Check sheet for the modelled part. Datum: model origin and axes. Units: mm. A direction names the side the tool comes from. Round coordinates to 2 decimals unless told otherwise and drop trailing zeros. Loops run counter-clockwise (first coordinate to the right, second up) from the corner with the lowest first, then second, coordinate; pieces in that order, holes last. Notation, with made-up numbers: (10.5, 48.5) -> (29.5, 48.5) arc R24 ccw to (29.5, 77.5) -> close; hole circle Ø9 at (31, 83). An arc over 180 degrees is marked (long way). Use one line per item in the form item = value. Start each with the question number.
(1) Go/stop test with flat-tipped pins: pin 1 (1.5 mm diameter, centred on x = -499, z = -663, fed in from +Y); pin 2 (2 mm diameter, centred on x = -357, y = 1222, fed in from +Z); pin 3 (12 mm diameter, centred on x = -530.68, z = -637.45, fed in from +Y); pin 4 (3 mm diameter, centred on x = -415, y = 993, fed in from -Z). Record where each tip stops, or that it passes through.
(2) Set-up check for faces 4 (the flat face through (-446, 1069, -657.097)), 5 (the cylindrical face through (-394.39, 1308.86, -642.06)), 6 (the flat face through (-486, 883, -732.097)), 7 (the flat face through (-404, 1075.621, -637)), 8 (the flat face through (-486, 873.179, -674)): record each of +Z, -Z, +X, -X, +Y, -Y from which the full face is reachable in a straight line by a thin tool's end or side.
(3) Sectioned sample at A-A (x = -366). Record the cut outline in (y, z).
(4) Draft check along X on faces 1 (the flat face through (-486, 893.179, -694)), 2 (the flat face through (-531, 926.127, -637)), 3 (the flat face through (-666.625, 1090, -641)). Enter one of: released by +X, released by -X, zero draft, split by the parting line, or undercut.
(5) Sectioned sample at B-B (y = 964.5). Record the cut outline in (x, z), and give its area (3 significant figures).
(6) Sectioned sample at C-C (y = 1179). Record the cut outline in (x, z), and give its area (3 significant figures).
(7) Sectioned sample at D-D (z = -634). Record the cut outline in (x, y).
(8) Material ranges on probe 1 along X at (y, z) = (1170.5, -637.5); probe 2 along Y at (x, z) = (-546, -626); probe 3 along X at (y, z) = (1058.5, -638), recorded low to high. Write a range as [from, to].
from build123d import *

# Parameters (mm, degrees)
SKETCH_1_W                      = 365.93
SKETCH_1_H                      = 455
SKETCH_1_R                      = 10
SKETCH_1_R_2                    = 14.438127561
SKETCH_1_W_2                    = 96.91
SKETCH_1_H_2                    = 352.59
SKETCH_1_H_3                    = 203.096012828
EXTRUDE_1_DEPTH                 = 40.26
CUT_EXTRUDE_1_REACH             = 1042.764
SKETCH_2_R                      = 10
CUT_EXTRUDE_1_DIRECTION_2_DEPTH = 1041.76399807
SKETCH_3_W                      = 365.93
SKETCH_3_H                      = 20
EXTRUDE_2_DEPTH                 = 80
CUT_EXTRUDE_2_REACH             = 1086.862
SKETCH_6_R                      = 12.5
CUT_EXTRUDE_4_DEPTH             = 1571.967331718
CUT_EXTRUDE_4_DEPTH_BACK        = 1571.967331718
SKETCH_9_W                      = 5
SKETCH_9_H                      = 20
CUT_EXTRUDE_5_DEPTH             = 1569.627549285
CUT_EXTRUDE_5_DEPTH_BACK        = 1569.627549285
SKETCH_10_W                     = 75
SKETCH_10_H                     = 10
SKETCH_11_W                     = 365.93
SKETCH_11_H                     = 115.26
SKETCH_11_R                     = 12.5
EXTRUDE_4_DEPTH                 = 10


with BuildPart() as part:
    # 草图1 → 凸台-拉伸1 (new body)
    with BuildSketch(Plane.XY.offset(-616.836895005)):
        with Locations((-483.659609698, 1110.678523142)):
            Rectangle(SKETCH_1_W, SKETCH_1_H)
        with Locations((-607.210787573, 1138.804962693)):
            Circle(SKETCH_1_R, mode=Mode.SUBTRACT)
        with Locations((-403.264609698, 1019.178523142)):
            Circle(SKETCH_1_R_2, mode=Mode.SUBTRACT)
        with Locations((-530.676153664, 1102.421638316)):
            Rectangle(SKETCH_1_W_2, SKETCH_1_H_2, mode=Mode.SUBTRACT)
        with Locations((-403.264609698, 1177.168631902)):
            Rectangle(SKETCH_1_W_2, SKETCH_1_H_3, mode=Mode.SUBTRACT)
    extrude(amount=-EXTRUDE_1_DEPTH)

    # 草图2 → 切除-拉伸1 (cut, up to next)
    with BuildSketch(Plane(origin=(0, 1338.178523142, 0), x_dir=(1, 0, 0), z_dir=(0, 1, 0)), mode=Mode.PRIVATE) as cut_extrude_1_sk1:
        with Locations(Location((-530.676153664, 637.446895005, 0), (0, 0, 90))):
            Circle(SKETCH_2_R)
    cut_extrude_1_tool1 = extrude(cut_extrude_1_sk1.sketch, amount=-CUT_EXTRUDE_1_REACH, mode=Mode.PRIVATE) & part.part
    # 草图2 → 切除-拉伸1 (cut, up to next)
    with BuildSketch(Plane(origin=(0, 1338.178523142, 0), x_dir=(1, 0, 0), z_dir=(0, 1, 0)), mode=Mode.PRIVATE) as cut_extrude_1_sk2:
        with Locations(Location((-403.264609698, 637.446895005, 0), (0, 0, 90))):
            Circle(SKETCH_2_R)
    cut_extrude_1_tool2 = extrude(cut_extrude_1_sk2.sketch, amount=-CUT_EXTRUDE_1_REACH, mode=Mode.PRIVATE) & part.part
    add(cut_extrude_1_tool1.solids().sort_by_distance((-530.676154, 1338.178523, -637.446895))[0], mode=Mode.SUBTRACT)
    add(cut_extrude_1_tool2.solids().sort_by_distance((-403.26461, 1338.178523, -637.446895))[0], mode=Mode.SUBTRACT)

    # 草图2 → 切除-拉伸1 direction 2 (cut)
    with BuildSketch(Plane(origin=(0, 1338.178523142, 0), x_dir=(1, 0, 0), z_dir=(0, 1, 0))):
        with Locations(Location((-530.676153664, 637.446895005, 0), (0, 0, 90))):
            Circle(SKETCH_2_R)
        with Locations(Location((-403.264609698, 637.446895005, 0), (0, 0, 90))):
            Circle(SKETCH_2_R)
    extrude(amount=CUT_EXTRUDE_1_DIRECTION_2_DEPTH, mode=Mode.SUBTRACT)

    # 草图3 → 凸台-拉伸2 (add)
    with BuildSketch(Plane(origin=(0, 0, -657.096895005), x_dir=(-1, 0, 0), z_dir=(0, 0, -1))):
        with Locations((483.659609698, 893.178523142)):
            Rectangle(SKETCH_3_W, SKETCH_3_H)
    extrude(amount=EXTRUDE_2_DEPTH)

    # 草图6 → 切除-拉伸2 (cut, up to next)
    with BuildSketch(Plane(origin=(0, 903.178523142, 0), x_dir=(1, 0, 0), z_dir=(0, 1, 0)), mode=Mode.PRIVATE) as cut_extrude_2_sk1:
        with Locations(Location((-566.624609698, 697.096895005, 0), (0, 0, 270))):
            Circle(SKETCH_6_R)
    cut_extrude_2_tool1 = extrude(cut_extrude_2_sk1.sketch, amount=-CUT_EXTRUDE_2_REACH, mode=Mode.PRIVATE) & part.part
    # 草图6 → 切除-拉伸2 (cut, up to next)
    with BuildSketch(Plane(origin=(0, 903.178523142, 0), x_dir=(1, 0, 0), z_dir=(0, 1, 0)), mode=Mode.PRIVATE) as cut_extrude_2_sk2:
        with Locations(Location((-400.694609698, 697.096895005, 0), (0, 0, 270))):
            Circle(SKETCH_6_R)
    cut_extrude_2_tool2 = extrude(cut_extrude_2_sk2.sketch, amount=-CUT_EXTRUDE_2_REACH, mode=Mode.PRIVATE) & part.part
    add(cut_extrude_2_tool1.solids().sort_by_distance((-566.62461, 903.178523, -697.096895))[0], mode=Mode.SUBTRACT)
    add(cut_extrude_2_tool2.solids().sort_by_distance((-400.69461, 903.178523, -697.096895))[0], mode=Mode.SUBTRACT)

    # 草图9 → 切除-拉伸4 (cut, two sides: drawn at the far end of the back side and taken through both)
    with BuildSketch(Plane(origin=(-300.694609698, 0, 0), x_dir=(0, 0, -1), z_dir=(1, 0, 0)).offset(-CUT_EXTRUDE_4_DEPTH_BACK)):
        with Locations((734.596895005, 893.178523142)):
            Rectangle(SKETCH_9_W, SKETCH_9_H)
    extrude(amount=CUT_EXTRUDE_4_DEPTH + CUT_EXTRUDE_4_DEPTH_BACK, mode=Mode.SUBTRACT)

    # 草图10 → 切除-拉伸5 (cut, two sides: drawn at the far end of the back side and taken through both)
    with BuildSketch(Plane(origin=(-300.694609698, 0, 0), x_dir=(0, 0, -1), z_dir=(1, 0, 0)).offset(-CUT_EXTRUDE_5_DEPTH_BACK)):
        with Locations((694.596895005, 898.178523142)):
            Rectangle(SKETCH_10_W, SKETCH_10_H)
    extrude(amount=CUT_EXTRUDE_5_DEPTH + CUT_EXTRUDE_5_DEPTH_BACK, mode=Mode.SUBTRACT)

    # 草图11 → 凸台-拉伸4 (add)
    with BuildSketch(Plane.XZ.offset(-883.178523142)):
        with Locations((-483.659609698, -674.466895005)):
            Rectangle(SKETCH_11_W, SKETCH_11_H)
        with Locations(Location((-400.694609698, -697.096895005, 0), (0, 0, 90))):
            Circle(SKETCH_11_R, mode=Mode.SUBTRACT)
        with Locations(Location((-566.624609698, -697.096895005, 0), (0, 0, 90))):
            Circle(SKETCH_11_R, mode=Mode.SUBTRACT)
    extrude(amount=EXTRUDE_4_DEPTH)


solid = part.part
Checks:
q1.pin_1 = 893.18
q1.pin_2 = through
q1.pin_3 = 926.13
q1.pin_4 = -657.1
q2.face_4 = -Z, +X, -X, +Y
q2.face_5 = +Y
q2.face_6 = -Z, +X, -X, +Y, -Y
q2.face_7 = +Z, -Z
q2.face_8 = +Z, -Z, +X, -X, -Y
q3.outline = (873.18, -732.1) -> (893.18, -732.1) -> (893.18, -657.1) -> (1075.62, -657.1) -> (1075.62, -616.84) -> (873.18, -616.84) -> close; (1278.72, -657.1) -> (1338.18, -657.1) -> (1338.18, -616.84) -> (1278.72, -616.84) -> close
q4.face_1 = zero draft
q4.face_2 = undercut
q4.face_3 = released by -X
q5.outline = (-666.62, -657.1) -> (-579.13, -657.1) -> (-579.13, -616.84) -> (-666.62, -616.84) -> close; (-482.22, -657.1) -> (-300.69, -657.1) -> (-300.69, -616.84) -> (-482.22, -616.84) -> close
q5.area = 10,800 mm2
q6.outline = (-666.62, -657.1) -> (-579.13, -657.1) -> (-579.13, -616.84) -> (-666.62, -616.84) -> close; (-482.22, -657.1) -> (-451.72, -657.1) -> (-451.72, -616.84) -> (-482.22, -616.84) -> close; (-354.81, -657.1) -> (-300.69, -657.1) -> (-300.69, -616.84) -> (-354.81, -616.84) -> close
q6.area = 6,930 mm2
q7.outline = (-666.62, 873.18) -> (-300.69, 873.18) -> (-300.69, 1338.18) -> (-393.88, 1338.18) -> (-393.88, 1278.72) -> (-354.81, 1278.72) -> (-354.81, 1075.62) -> (-451.72, 1075.62) -> (-451.72, 1278.72) -> (-412.65, 1278.72) -> (-412.65, 1338.18) -> (-521.29, 1338.18) -> (-521.29, 1278.72) -> (-482.22, 1278.72) -> (-482.22, 926.13) -> (-579.13, 926.13) -> (-579.13, 1278.72) -> (-540.06, 1278.72) -> (-540.06, 1338.18) -> (-666.62, 1338.18) -> close; hole circle Ø20 at (-607.21, 1138.8); hole circle Ø28.88 at (-403.26, 1019.18)
q8.probe_1 = [-666.62, -579.13], [-482.22, -451.72], [-354.81, -300.69]
q8.probe_2 = [873.18, 926.13], [1278.72, 1338.18]
q8.probe_3 = [-666.62, -579.13], [-482.22, -300.69]
